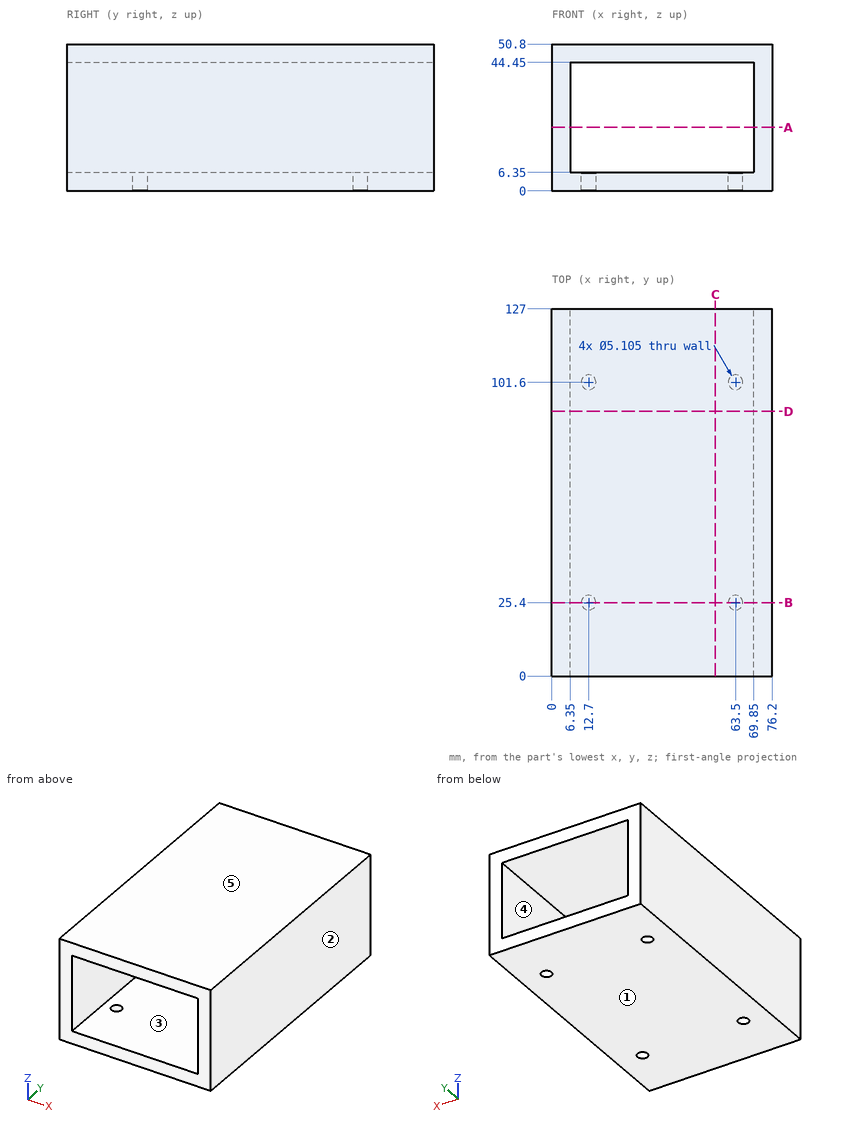
Answer from the drawing. Dimensions are ordinates in mm from the lowest x, y and z of the part. A direction names the side the tool comes from. Coordinates: 2 decimals unless noted, no trailing zeros. Write each loop counter-clockwise with the first axis right and the second up, starting at its lowest first coordinate (ties: lowest second). Pieces come first, ordered by that corner, then holes. Notation, with made-up numbers: M -3,72 L 56,72 A21 ccw 56,80 Z; hole C -11.75,27.25 d5. An arc over 180 degrees is marked long. Put each result on its own line as item: value. Start each with the question number.
1. A cutting plane is placed at A-A on z = 22. Write down the section's boundary in (x, y), then the cut area to 3 significant figures.
2. Which of the six approach directions +Z, -Z, +X, -X, +Y, -Y give full straight-line access (tool end or side, diameter ignored) to the marked faces 4 and 5?
3. For a pull along X with two mould halves and no side action, classify the marked faces 1, 2 and 3 as pulls with the +X half, pulls with the -X half, needs draft (parallel to the pull), parting line crosses it, or undercut.
4. A cutting plane is placed at C-C on x = 56.5. Write down the section's boundary in (y, z), then the cut area to 3 significant figures.
5. A cutting plane is placed at D-D on y = 91.5. Write down the section's boundary in (x, z), then the cut area to 3 significant figures.
6. Flat-ended cylindrical pins translate along their axes: P1, Ø5, axis at x = 37, y = 79, coming from the -Z side; P2, Ø4, axis at x = 12.7, y = 101.6, coming from the -Z side. Find the tip coordinate at first contact, or state that the pin passes through.
7. A cutting plane is placed at B-B on y = 25.4. Write down the section's boundary in (x, z).
8. Consider line 1 (Y direction, x = 12.7, z = 5.25); line 2 (X direction, y = 108.5, z = 15); line 3 (Z direction, x = 17, y = 42). Determine where each line is inside the solid, lowest interval first. Write a range as from..to.
Resolved:
1. outline: M 0,0 L 6.35,0 L 6.35,127 L 0,127 Z; M 69.85,0 L 76.2,0 L 76.2,127 L 69.85,127 Z
1. area: 1,610 mm2
2. face 4: +Y, -Y
2. face 5: +Z, +X, -X, +Y, -Y
3. face 1: needs draft
3. face 2: pulls with the +X half
3. face 3: undercut
4. outline: M 0,0 L 127,0 L 127,6.35 L 0,6.35 Z; M 0,44.45 L 127,44.45 L 127,50.8 L 0,50.8 Z
4. area: 1,610 mm2
5. outline: M 0,0 L 76.2,0 L 76.2,50.8 L 0,50.8 Z; hole M 6.35,6.35 L 69.85,6.35 L 69.85,44.45 L 6.35,44.45 Z
5. area: 1,450 mm2
6. P1: stops at z = 0
6. P2: stops at z = 44.45
7. outline: M 0,0 L 10.15,0 L 10.15,6.35 L 6.35,6.35 L 6.35,44.45 L 69.85,44.45 L 69.85,6.35 L 66.05,6.35 L 66.05,0 L 76.2,0 L 76.2,50.8 L 0,50.8 Z; M 15.25,0 L 60.95,0 L 60.95,6.35 L 15.25,6.35 Z
8. line 1: y = 0..22.85, 27.95..99.05, 104.15..127
8. line 2: x = 0..6.35, 69.85..76.2
8. line 3: z = 0..6.35, 44.45..50.8
